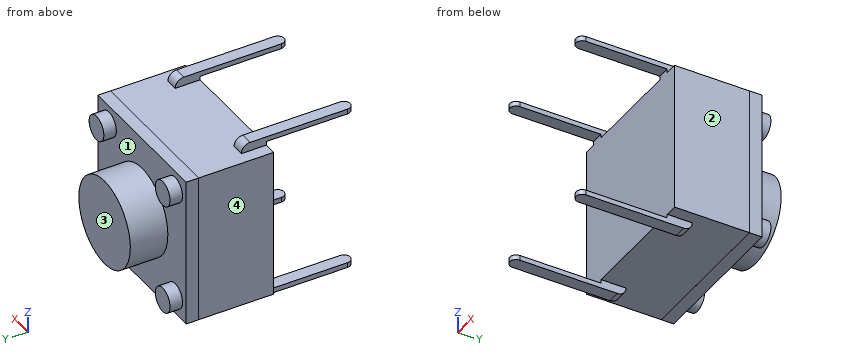
```python
from build123d import *

# Parameters (mm, degrees)
CROQUIS3_W               = 6
CROQUIS3_H               = 6
SALIENTE_EXTRUIR4_DEPTH  = 3
CROQUIS6_W               = 6.001
CROQUIS6_H               = 6.001
SALIENTE_EXTRUIR9_DEPTH  = 0.5
CROQUIS7_R               = 0.5
SALIENTE_EXTRUIR10_DEPTH = 0.5
CROQUIS7_3_R             = 1.75
SALIENTE_EXTRUIR11_DEPTH = 1.5
SALIENTE_EXTRUIR12_DEPTH = 0.35
REDONDEO3_R              = 0.35
REDONDEO3_OF_SIMETR_A4_R = 0.35
CROQUIS11_W              = 6
CROQUIS11_H              = 6.3
CORTAR_EXTRUIR1_DEPTH    = 6.2


with BuildPart() as part:
    # Croquis3 → Saliente-Extruir4 (new body)
    with BuildSketch(Plane(origin=(0, 0, 0), x_dir=(1, 0, 0), z_dir=(0, 1, 0))):
        Rectangle(CROQUIS3_W, CROQUIS3_H)
    extrude(amount=SALIENTE_EXTRUIR4_DEPTH)

    # Croquis6 → Saliente-Extruir9 (add)
    with BuildSketch(Plane(origin=(0, 3, 0), x_dir=(1, 0, 0), z_dir=(0, 1, 0))):
        Rectangle(CROQUIS6_W, CROQUIS6_H)
    extrude(amount=SALIENTE_EXTRUIR9_DEPTH)

    # Croquis7 → Saliente-Extruir10 (add)
    with BuildSketch(Plane(origin=(0, 3.5, 0), x_dir=(1, 0, 0), z_dir=(0, 1, 0))):
        with Locations(Location((-2.25, -2.25, 0), (0, 0, 270))):
            Circle(CROQUIS7_R)
        with Locations(Location((-2.25, 2.25, 0), (0, 0, 270))):
            Circle(CROQUIS7_R)
        with Locations(Location((2.25, 2.25, 0), (0, 0, 270))):
            Circle(CROQUIS7_R)
        with Locations(Location((2.25, -2.25, 0), (0, 0, 270))):
            Circle(CROQUIS7_R)
    extrude(amount=SALIENTE_EXTRUIR10_DEPTH)

    # Croquis7<3> → Saliente-Extruir11 (add)
    with BuildSketch(Plane(origin=(0, 3.5, 0), x_dir=(1, 0, 0), z_dir=(0, 1, 0))):
        with Locations(Location((0, 0, 0), (0, 0, 270))):
            Circle(CROQUIS7_3_R)
    extrude(amount=SALIENTE_EXTRUIR11_DEPTH)

    # Croquis8 → Saliente-Extruir12 (add)
    with BuildSketch(Plane.XY.offset(3)):
        with BuildLine():
            Line((-2.5, 1), (-2, 1))
            Line((-2, 1), (-2, -3.25))
            ThreePointArc((-2, -3.25), (-2.25, -3.5), (-2.5, -3.25))
            Line((-2.5, -3.25), (-2.5, 1))
        make_face()
        with BuildLine():
            Line((2, 1), (2, -3.25))
            ThreePointArc((2, -3.25), (2.25, -3.5), (2.5, -3.25))
            Line((2.5, -3.25), (2.5, 1))
            Line((2.5, 1), (2, 1))
        make_face()
    saliente_extruir12 = extrude(amount=SALIENTE_EXTRUIR12_DEPTH)

    # Redondeo3
    redondeo3_edges = [part.edges().sort_by_distance(p)[0] for p in [
        (-2.25, 1, 3.35),
        (2.25, 1, 3.35),
    ]]
    fillet(redondeo3_edges, radius=REDONDEO3_R - 0.0001)  # a hair under: the kernel refuses the full size

    # Simetría4: Saliente-Extruir12 across plane
    add(saliente_extruir12.mirror(Plane.XY))

    # Redondeo3 of Simetría4
    redondeo3_of_simetr_a4_edges = [part.edges().sort_by_distance(p)[0] for p in [
        (-2.25, 1, -3.35),
        (2.25, 1, -3.35),
    ]]
    fillet(redondeo3_of_simetr_a4_edges, radius=REDONDEO3_OF_SIMETR_A4_R - 0.0001)  # a hair under: the kernel refuses the full size

    # Croquis11 → Cortar-Extruir1 (cut)
    with BuildSketch(Plane.XZ):
        Rectangle(CROQUIS11_W, CROQUIS11_H)
    extrude(amount=CORTAR_EXTRUIR1_DEPTH, mode=Mode.SUBTRACT)


solid = part.part
```
Geometry check sheet. Reference: the model listing, model coordinates, mm. Face numbers are marked on the shaded views. Coordinates: 2 decimals unless noted, no trailing zeros. Order: outer loops, then holes, each group sorted by start corner. A loop starts at its lowest first (then second) coordinate and runs counter-clockwise, first axis right, second up.
Q1. Depth check by flat-ended pin: pin 1 Ø2 at (x, z) = (-1.5, 1.5) entering from -Y; pin 2 Ø2 at (x, y) = (-1.5, 2) entering from +Z; pin 3 Ø1.1 at (x, z) = (-2, 2) entering from +Y. Enter the tip coordinate at first touch or a pass-through.
Reply:
pin 1: stops at y = 0
pin 2: stops at z = 3
pin 3: stops at y = 4
Q2. Draft check along X on the marked faces 1, 2, 3 and 4. Enter one of: released by +X, released by -X, zero draft, split by the parting line, or undercut.
Reply:
face 1: undercut
face 2: released by +X
face 3: zero draft
face 4: released by -X
Q3. Sectioned sample at B-B on y = -0.5. Record the cut outline in (x, z), and give its area (3 significant figures).
Reply:
outline: (-2.5, -3.35) - (-2, -3.35) - (-2, -3.15) - (-2.5, -3.15) - close; (-2.5, 3.15) - (-2, 3.15) - (-2, 3.35) - (-2.5, 3.35) - close; (2, -3.35) - (2.5, -3.35) - (2.5, -3.15) - (2, -3.15) - close; (2, 3.15) - (2.5, 3.15) - (2.5, 3.35) - (2, 3.35) - close
area: 0.400 mm2
Q4. Thickness scan on probe 1 along Y at (x, z) = (1.5, 1); probe 2 along Z at (x, y) = (2.25, -0.25); probe 3 along Y at (x, z) = (-2.25, 2.5). Record the ranges inside material, lowest first.
Reply:
probe 1: y = 0 to 3.5
probe 2: z = -3.35 to -3.15, 3.15 to 3.35
probe 3: y = 0 to 4
